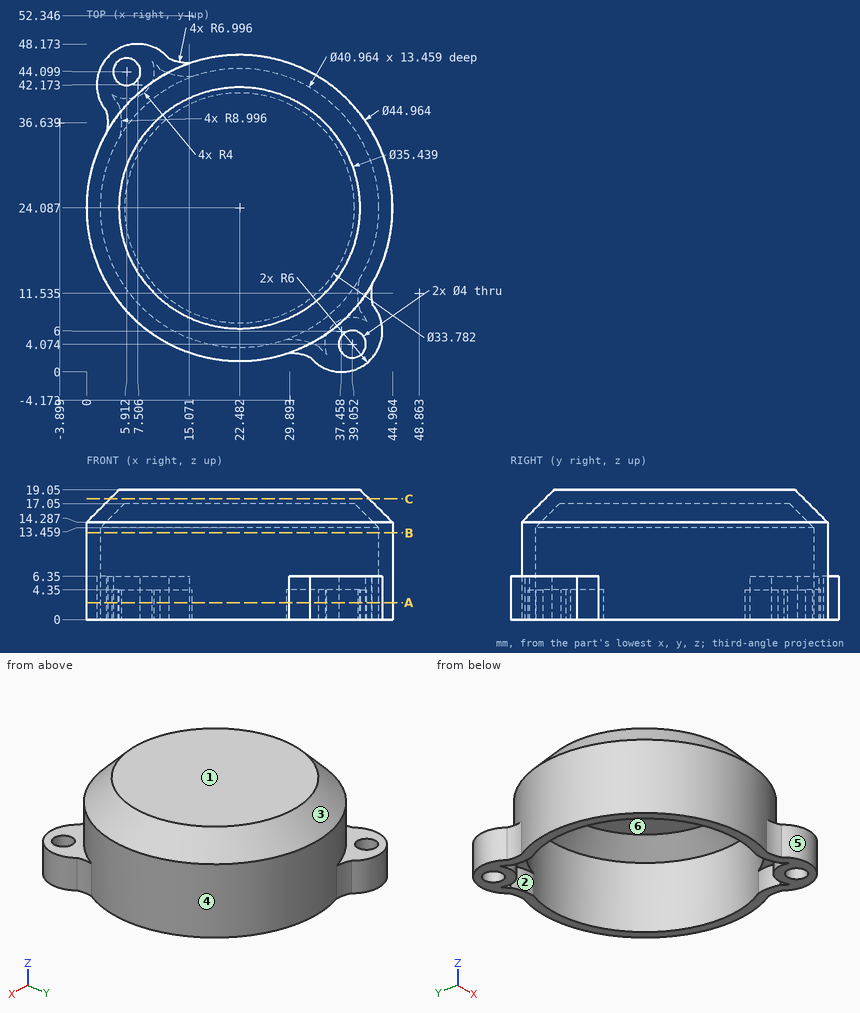
The figure shows three views and two pictorial views of one solid part (mm, origin at its lowest corner). Answer the questions. A direction names the side the tool comes from. Round coordinates to 2 decimals unless told otherwise and drop trailing zeros. Loops run counter-clockwise (first coordinate to the right, second up) from the corner with the lowest first, then second, coordinate; pieces in that order, holes last. Notation, with made-up numbers: M 69,85 L 108,85 A26 cw 108,114 Z; hole C -13.75,54.5 d2. An arc over 180 degrees is marked long. Write each question's results on one line, items separated by ' | '. Start each with the question number.
1) Determine the mould class of the marked faces 1, 2 and 3 for opening direction X: pulls with the +X half, pulls with the -X half, needs draft (parallel to the pull), parting line crosses it, or undercut.
2) Straight lines are drawn through the part: probe 1 along Z at (x, y) = (18.5, 23.5); probe 2 along X at (y, z) = (23, 3.5) (1 decimal); probe 3 along X at (y, z) = (15.5, 6.25) (1 decimal). For each, find the intervals that lie inside material, in ascending order.
3) Find section C-C on z = 17.75. Write down the section's boundary in (x, y), plus the area to 3 significant figures.
4) Find section B-B on z = 12.75. Write down the section's boundary in (x, y) (1 decimal), plus the area to 3 significant figures.
5) Each of these flat-tipped pins is pushed along its axis until it touches: pin 1 (10.5 mm diameter, centred on x = 35, y = 4, fed in from +Z); pin 2 (5.5 mm diameter, centred on x = 33.5, y = 6.5, fed in from -Z); pin 3 (6.5 mm diameter, centred on x = 6.5, y = 40, fed in from +Z) (1 decimal); pin 4 (6 mm diameter, centred on x = 35.5, z = 10.5, fed in from -Y). Where does it stop, or does it pass through?
6) Which of the six approach directions +Z, -Z, +X, -X, +Y, -Y give full straight-line access (tool end or side, diameter ignored) to the marked faces 4, 5 and 6?
7) Find section A-A on z = 2.5. Count the separate pieces of the cut face and the enclosed holes in it.
Final values:
1) face 1: needs draft | face 2: undercut | face 3: parting line crosses it
2) probe 1: 17.05 to 19.05 | probe 2: 0 to 2, 42.9 to 44.9 | probe 3: 1.7 to 3.9, 41.1 to 43.3
3) outline: C 22.48,24.09 d38.04 | area: 1,140 mm²
4) outline: C 22.5,24.1 d45; hole C 22.5,24.1 d41 | area: 270 mm²
5) pin 1: z = 18.35 | pin 2: z = 0 | pin 3: z = 17.5 | pin 4: y = 3.96
6) face 4: +Z | face 5: +Z, -Z | face 6: -Z
7) separate pieces: 1 | enclosed holes: 3
